Input: part model. Units: mm. Frame: model coordinates. Face numbers are marked on the shaded views. A direction names the side the tool comes from. Coordinates: 2 decimals unless noted, no trailing zeros. Write each loop counter-clockwise with the first axis right and the second up, starting at its lowest first coordinate (ties: lowest second). Pieces come first, ordered by that corner, then holes.
1) Section query A-A (y = -37.5). Output: boundary loops of the cut face in (x, z), then the cut area to 3 significant figures.
2) Section query C-C (z = 15). Output: boundary loops of the cut face in (x, y).
3) Line query: L1, parallel to Y at x = -39.5, z = 7; L2, parallel to X at y = -31, z = 13.5; L3, parallel to Y at x = -39, z = 8. Output: solid intervals per line, ascending.
4) Section query B-B (x = 39.5). Output: boundary loops of the cut face in (y, z), then the cut area to 3 significant figures.
5) Set-up query: the marked faces 5, 6, 7, 8 and 9. Return all of +Z, -Z, +X, -X, +Y, -Y with unobstructed straight access to the full face (end or side cutting, diameter ignored); none if empty.
6) Draft query along X for the marked faces 1, 2, 3 and 4. Return one class per face: pulls with the +X half, pulls with the -X half, needs draft (parallel to the pull), parting line crosses it, or undercut.
7) Section query D-D (x = -20). Output: boundary loops of the cut face in (y, z), then the cut area to 3 significant figures.
8) Pin query (flat end, axial travel): pin 1 Ø2.5 at (x, z) = (27, 22.5) entering from +Y; pin 2 Ø5 at (x, y) = (-4, -31) entering from -Z; pin 3 Ø6.5 at (x, y) = (-39.5, 6.92) entering from +Z; pin 4 Ø2.5 at (x, z) = (-28.5, 47.5) entering from +Y. Return the tip coordinate at first contact, or that it passes through.
from build123d import *

# Parameters (mm, degrees)
SKETCH1_R             = 2
BOSS_EXTRUDE2_DEPTH   = 10
BOSS_EXTRUDE2_2_DEPTH = 10
BOSS_EXTRUDE2_3_DEPTH = 10
SKETCH1_8_W           = 8
SKETCH1_8_H           = 41
BOSS_EXTRUDE3_DEPTH   = 60
CUT_EXTRUDE1_REACH    = 111.65
FILLET3_R             = 20
FILLET4_R             = 10
FILLET5_R             = 20
SKETCH3_R             = 1.6
CUT_EXTRUDE3_DEPTH    = 96.421433651


with BuildPart() as part:
    # Sketch1 → Boss-Extrude2 (new body)
    with BuildSketch(Plane.XY):
        with BuildLine():
            Line((-47.5, 20.92242842), (-47.5, -36.07757158))
            Line((-47.5, -36.07757158), (-47.5, -44.07757158))
            Line((-47.5, -44.07757158), (-33, -44.07757158))
            Line((-33, -44.07757158), (-33, -36.07757158))
            Line((-33, -36.07757158), (-33, 4.92242842))
            Line((-33, 4.92242842), (-25, 4.92242842))
            ThreePointArc((-25, 4.92242842), (-24.979959865, 5.923230668), (-24.919871589, 6.92242842))
            Line((-24.919871589, 6.92242842), (-25, 20.92242842))
            Line((-25, 20.92242842), (-47.5, 20.92242842))
        make_face()
        with Locations((-39.5, 0.92242842)):
            Circle(SKETCH1_R, mode=Mode.SUBTRACT)
        with Locations((-39.5, 6.92242842)):
            Circle(SKETCH1_R, mode=Mode.SUBTRACT)
        with Locations((-39.5, 12.92242842)):
            Circle(SKETCH1_R, mode=Mode.SUBTRACT)
    extrude(amount=BOSS_EXTRUDE2_DEPTH)



with BuildPart() as body_2:
    # Sketch1 → Boss-Extrude2 2 (new body)
    with BuildSketch(Plane.XY):
        with BuildLine():
            ThreePointArc((24.677925359, 0.92242842), (-2.00647278, -19.996922835), (-25, 4.92242842))
            Line((-25, 4.92242842), (-25, -36.07757158))
            Line((-25, -36.07757158), (0, -36.07757158))
            Line((0, -36.07757158), (25, -36.07757158))
            Line((25, -36.07757158), (25, 4.92242842))
            ThreePointArc((25, 4.92242842), (24.919351255, 2.915955639), (24.677925359, 0.92242842))
        make_face()
    extrude(amount=BOSS_EXTRUDE2_2_DEPTH)


with BuildPart() as body_3:
    # Sketch1 → Boss-Extrude2 3 (new body)
    with BuildSketch(Plane.XY):
        with BuildLine():
            Line((33, -36.07757158), (33, -44.07757158))
            Line((33, -44.07757158), (47.5, -44.07757158))
            Line((47.5, -44.07757158), (47.5, -36.07757158))
            Line((47.5, -36.07757158), (47.5, 20.92242842))
            Line((47.5, 20.92242842), (25, 20.92242842))
            Line((25, 20.92242842), (24.919871589, 6.92242842))
            ThreePointArc((24.919871589, 6.92242842), (24.979959865, 5.923230668), (25, 4.92242842))
            Line((25, 4.92242842), (33, 4.92242842))
            Line((33, 4.92242842), (33, -36.07757158))
        make_face()
        with Locations((39.5, 0.92242842)):
            Circle(SKETCH1_R, mode=Mode.SUBTRACT)
        with Locations((39.5, 6.92242842)):
            Circle(SKETCH1_R, mode=Mode.SUBTRACT)
        with Locations((39.5, 12.92242842)):
            Circle(SKETCH1_R, mode=Mode.SUBTRACT)
    extrude(amount=BOSS_EXTRUDE2_3_DEPTH)


with BuildPart() as part_1:
    add(part.part)

    add(body_2.part)  # Boss-Extrude3 merges body 2

    add(body_3.part)  # Boss-Extrude3 merges body 3
    # Sketch1_8 → Boss-Extrude3 (add)
    with BuildSketch(Plane.XY):
        with Locations((-29, -15.57757158)):
            Rectangle(SKETCH1_8_W, SKETCH1_8_H)
        Polygon((-33, -36.07757158), (-33, -44.07757158), (33, -44.07757158), (33, -36.07757158), (25, -36.07757158), (0, -36.07757158), (-25, -36.07757158), align=None)
        with Locations((29, -15.57757158)):
            Rectangle(SKETCH1_8_W, SKETCH1_8_H)
    extrude(amount=BOSS_EXTRUDE3_DEPTH)

    # Sketch2 → Cut-Extrude1 (cut, up to next)
    with BuildSketch(Plane.ZY.offset(33), mode=Mode.PRIVATE) as cut_extrude1_sk1:
        Polygon((41.60617838, -22.329937261), (41.60617838, 4.92242842), (60, 4.92242842), (60, -36.07757158), (55.59382162, -36.025205899), (41.60617838, -36.025205899), align=None)
    cut_extrude1_tool1 = extrude(cut_extrude1_sk1.sketch, amount=-CUT_EXTRUDE1_REACH, mode=Mode.PRIVATE) & part_1.part
    add(cut_extrude1_tool1.solids().sort_by_distance((-33, -15.554527, 50.804273))[0], mode=Mode.SUBTRACT)

    # Fillet3
    fillet3_edges = [part_1.edges().sort_by_distance(p)[0] for p in [
        (29, 4.92242842, 60),
    ]]
    fillet(fillet3_edges, radius=FILLET3_R)

    # Fillet4
    fillet4_edges = [part_1.edges().sort_by_distance(p)[0] for p in [
        (-25, 20.92242842, 5),
        (25, 20.92242842, 5),
    ]]
    fillet(fillet4_edges, radius=FILLET4_R)

    # Fillet5
    fillet5_edges = [part_1.edges().sort_by_distance(p)[0] for p in [
        (-29, 4.92242842, 41.60617838),
    ]]
    fillet(fillet5_edges, radius=FILLET5_R)

    # Sketch3 → Cut-Extrude3 (cut, through all)
    with BuildSketch(Plane(origin=(0, -36.07757158, 0), x_dir=(1, 0, 0), z_dir=(0, 1, 0))):
        with Locations(Location((-20, -55, 0), (0, 0, 270))):
            Circle(SKETCH3_R)
        with Locations(Location((20, -15, 0), (0, 0, 270))):
            Circle(SKETCH3_R)
    extrude(amount=-CUT_EXTRUDE3_DEPTH, mode=Mode.SUBTRACT)


solid = part_1.part
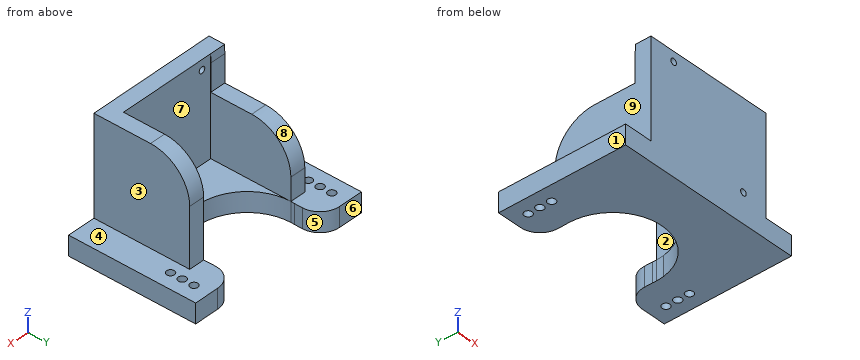
Answer:
1. outline: (-47.5, 0) - (47.5, 0) - (47.5, 10) - (33, 10) - (33, 60) - (-33, 60) - (-33, 10) - (-47.5, 10) - close; hole circle Ø3.2 at (-20, 55); hole circle Ø3.2 at (20, 15)
1. area: 4,230 mm2
2. outline: (-33, -44.08) - (18.4, -44.08) - (18.4, -36.08) - (-25, -36.08) - (-25, 4.92) - (-33, 4.92) - close; (21.6, -44.08) - (33, -44.08) - (33, 4.92) - (25, 4.92) - (25, -36.08) - (21.6, -36.08) - close
3. L1: y = -44.08 to -1.08, 2.92 to 4.92, 8.92 to 10.92, 14.92 to 20.92
3. L2: x = -33 to -25, 25 to 33
3. L3: y = -44.08 to -1.01, 2.86 to 4.99, 8.86 to 10.99, 14.86 to 20.92
4. outline: (-44.08, 0) - (-1.08, 0) - (-1.08, 10) - (-44.08, 10) - close; (2.92, 0) - (4.92, 0) - (4.92, 10) - (2.92, 10) - close; (8.92, 0) - (10.92, 0) - (10.92, 10) - (8.92, 10) - close; (14.92, 0) - (20.92, 0) - (20.92, 10) - (14.92, 10) - close
4. area: 530 mm2
5. face 5: +Z, -Z, +Y
5. face 6: +Z, -Z, +X, -X, +Y
5. face 7: +Z, +Y
5. face 8: +Z, -X, +Y
5. face 9: +Z, -X, +Y, -Y
6. face 1: pulls with the -X half
6. face 2: undercut
6. face 3: pulls with the +X half
6. face 4: needs draft
7. outline: (-44.08, 0) - (-10.08, 0) - (-10.08, 10) - (-36.08, 10) - (-36.08, 53.4) - (-44.08, 53.4) - close; (-44.08, 56.6) - (-36.08, 56.6) - (-36.08, 60) - (-44.08, 60) - close
7. area: 714 mm2
8. pin 1: stops at y = 4.92
8. pin 2: stops at z = 0
8. pin 3: stops at z = 10
8. pin 4: stops at y = -36.03
